Autodesk Inventor part; units mm, degrees
ref_plane "YZ Plane" through (0, 0, 0) normal (1, 0, 0) x (0, 1, 0)
ref_plane "XZ Plane" through (0, 0, 0) normal (0, 1, 0) x (-1, 0, 0)
ref_plane "XY Plane" through (0, 0, 0) normal (0, 0, 1) x (1, 0, 0)
sketch "Sketch1" plane through (0, 0, 0) normal (0, 0, 1) x (1, 0, 0)
  circle A0 centre (0, 0) radius 2.5
  line L0 (2, 1.5) -> (2, -1.5)
  dimension "d0" = 5
  dimension "d1" = 2
extrude "Extrusion1" add sketch "Sketch1" against normal blind 52
extrude "Extrusion2" cut sketch "Sketch1" against normal blind 10 contours A0 L0 picked at (2.0912, -0.3466)
chamfer "Chamfer1" distance 0.5 angle 45 2 edges at (-2.5, 0, 0) (-2.5, 0, -52)
properties part number "Flywheelshaft"
Source: CAD feature listing. Evaluate the final solid. Frame: model axes, mm. A direction names the side the tool comes from. Round coordinates to 2 decimals unless told otherwise and drop trailing zeros. Write each loop counter-clockwise with the first axis right and the second up, starting at its lowest first coordinate (ties: lowest second). Pieces come first, ordered by that corner, then holes. Notation, with made-up numbers: M 14,39 L 27,39 A9 cw 27,50 Z; hole C 49.5,47 d1. An arc over 180 degrees is marked long. Use CSV: the item, a comma, the result in double quotes. Start each with the question number.
Q1. First-contact query: P1, Ø1.5, axis at y = 0, z = -7, coming from the +X side; P2, Ø1, axis at x = -1, z = -20.5, coming from the +Y side; P3, Ø3, axis at y = -2, z = -19, coming from the +X side. Flat tips, straight axial feed; report the tip coordinate or a pass-through.
Q2. Access query for faces 1 (the face through (2, 0, -5)), 2 (the face through (0, 0, 0)). Directions: +Z, -Z, +X, -X, +Y, -Y. A direction counts if a zero-diameter tool reaches every point of the face in a straight line with its end or side. Return the directions, or none.
Q3. Cut plane B-B on z = -14. Output: boundary loops of the cut face in (x, y), plus the area to 3 significant figures.
Q4. Cut plane A-A on y = 0. Output: boundary loops of the cut face in (x, z).
Q5. Line query: line 1 (X direction, y = 1.5, z = -49); line 2 (X direction, y = 0.1, z = -13); line 3 (Y direction, x = 1.7, z = -43). Output: solid intervals per line, ascending. Write a range as from..to.
Results found:
1,P1,"x = 2"
1,P2,"y = 2.45"
1,P3,"x = 2.45"
2,face 1,"+Z, +X, +Y, -Y"
2,face 2,"+Z, +X, -X, +Y, -Y"
3,outline,"C 0,0 d5"
3,area,"19.6 mm^2"
4,outline,"M -2.5,-51.5 L -2,-52 L 2,-52 L 2.5,-51.5 L 2.5,-10 L 2,-10 L 2,0 L -2,0 L -2.5,-0.5 Z"
5,line 1,"-2..2"
5,line 2,"-2.5..2.5"
5,line 3,"-1.83..1.83"
